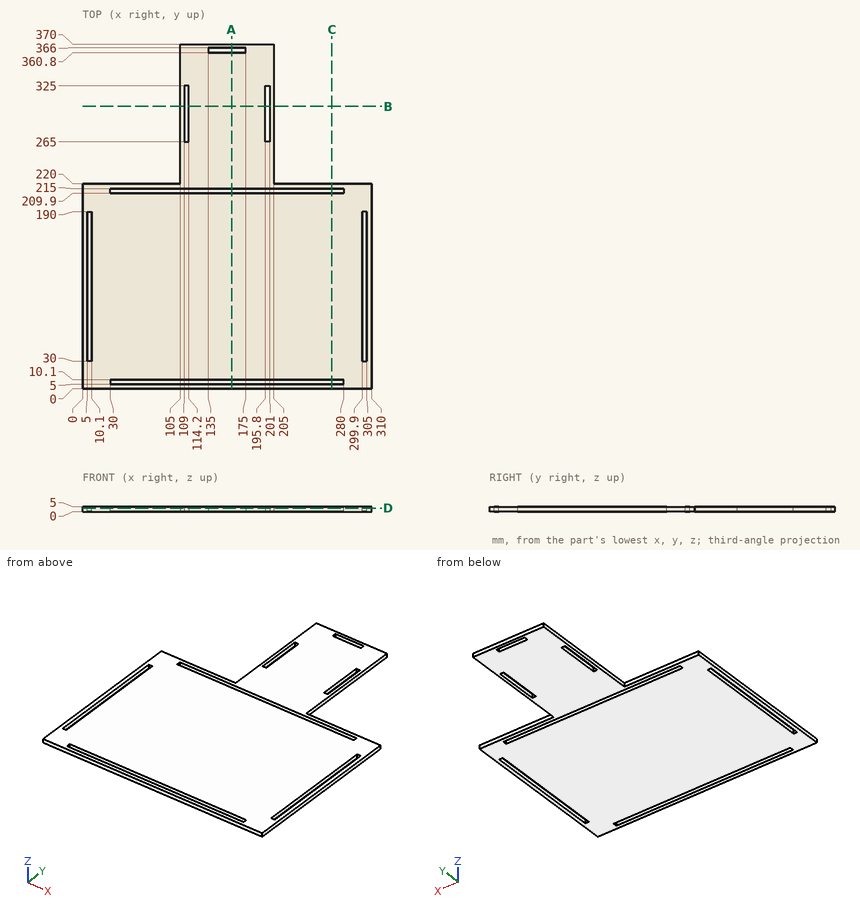
Could you check a few things on this drawing? It's one solid part, dimensions in mm from its lowest x, y, z. Round coordinates to 2 decimals unless told otherwise and drop trailing zeros. Write each loop counter-clockwise with the first axis right and the second up, starting at its lowest first coordinate (ties: lowest second). Pieces come first, ordered by that corner, then holes. Notation, with made-up numbers: (-24.75, -35) -> (8.25, -35) arc R14 ccw to (8.25, -18) -> close; hole circle Ø5 at (33.5, 33.5). An arc over 180 degrees is marked (long way). Use a Markdown table: item, result.
1. If we section it at B-B (y = 303): List the corners of the cut face in (x, z) for me, then the cut area to 3 significant figures.
Answer key:
| item | result |
|---|---|
| outline | (105, 0) -> (109, 0) -> (109, 5) -> (105, 5) -> close; (114.2, 0) -> (195.8, 0) -> (195.8, 5) -> (114.2, 5) -> close; (201, 0) -> (205, 0) -> (205, 5) -> (201, 5) -> close |
| area | 448 mm^2 |
2. If we section it at A-A (x = 160): List the corners of the cut face in (y, z) for me, then the cut area to 3 significant figures.
Answer key:
| item | result |
|---|---|
| outline | (0, 0) -> (5, 0) -> (5, 5) -> (0, 5) -> close; (10.1, 0) -> (209.9, 0) -> (209.9, 5) -> (10.1, 5) -> close; (215, 0) -> (360.8, 0) -> (360.8, 5) -> (215, 5) -> close; (366, 0) -> (370, 0) -> (370, 5) -> (366, 5) -> close |
| area | 1,770 mm^2 |
3. If we section it at C-C (x = 267.5): List the corners of the cut face in (y, z) for me.
Answer key:
| item | result |
|---|---|
| outline | (0, 0) -> (5, 0) -> (5, 5) -> (0, 5) -> close; (10.1, 0) -> (209.9, 0) -> (209.9, 5) -> (10.1, 5) -> close; (215, 0) -> (220, 0) -> (220, 5) -> (215, 5) -> close |
4. If we section it at D-D (z = 3.65): State how many separate pieces and enclosed holes the cut face has, then the cut area to 3 significant figures.
Answer key:
| item | result |
|---|---|
| separate pieces | 1 |
| enclosed holes | 7 |
| area | 78,200 mm^2 |
5. For pin 1 Ø1 at (x, z) = (195, 2) entering from -Y; pin 2 Ø2.5 at (y, z) = (299.5, 2) entering from +X; pin 3 Ø1.5 at (y, z) = (323, 2.5) entering from -X, each with a flat end and sliding along its axis, tell me the tip position at first contact or that it passes through.
Answer key:
| item | result |
|---|---|
| pin 1 | stops at y = 0 |
| pin 2 | stops at x = 205 |
| pin 3 | stops at x = 105 |
6. Please list where these lines run through material, in increasing order: probe 1 along Y at (x, z) = (183.5, 4.8); probe 2 along Y at (x, z) = (161, 3.05); probe 3 along X at (y, z) = (303, 0.3).
Answer key:
| item | result |
|---|---|
| probe 1 | y = 0 to 5, 10.1 to 209.9, 215 to 370 |
| probe 2 | y = 0 to 5, 10.1 to 209.9, 215 to 360.8, 366 to 370 |
| probe 3 | x = 105 to 109, 114.2 to 195.8, 201 to 205 |
